The listing builds one solid part. Answer for the finished solid, in the listing's coordinates (mm). A direction names the side the tool comes from. Round coordinates to 2 decimals unless told otherwise and drop trailing zeros. Order: outer loops, then holes, each group sorted by start corner. A loop starts at its lowest first (then second) coordinate and runs counter-clockwise, first axis right, second up. Notation, with made-up numbers: (-22.5, -10) - (-12.5, -10) arc R21 ccw to (-12.5, -6) - close; hole circle Ø6 at (-17.75, -18.75). An arc over 180 degrees is marked (long way). Use CSV: the item, a comma, the result in double quotes. Start each with the question number.
Item 1: Flat-ended cylindrical pins translate along their axes: P1, Ø2, axis at y = 5.5, z = 35.5, coming from the +X side (3 decimals); P2, Ø3.5, axis at y = 0, z = -19.05, coming from the +X side. Find the tip coordinate at first contact, or state that the pin passes through.
Item 2: Determine the mould class of faces 1 (the flat face through (-13, 12.7, 20)), 2 (the flat face through (-20.32, 0, 18)), 3 (the conical face through (-18.66, -0.13, 33.97)), 4 (the flat face through (-13, -12.7, 20)) for opening direction Y: +Y half, -Y half, draft (parallel to the pull), parting line (faces both ways), or undercut.
Item 3: Find section D-D, the plane z = 48.5. Give the vertices of the cut face in (x, y) (3 decimals), plus the area to 3 significant figures.
Item 4: Straight lines are drawn through the part: line 1 along Z through (x, y) = (-12.25, 0); line 2 along Z through (x, y) = (-5.75, 0); line 3 along Z through (x, y) = (-7, 0). For each, find the intervals that lie inside material, in ascending order. Write a range as [from, to].
Item 5: For faces 5 (the flat face through (-3.175, 0, 44)), 6 (the cylindrical face through (-10.515, 0.607, 36.216)), 7 (the flat face through (-11, 0, -25.4)), determine the directions among +Z, -Z, +X, -X, +Y, -Y from which every point of the face is accessible in a straight line to the end or side of a thin tool.
Item 6: Find section B-B, the plane y = -4.25. Give the vertices of the cut face in (x, z) (3 decimals), plus the area to 3 significant figures.
Item 7: Find section C-C, the plane x = -8.75. Give the vertices of the cut face in (y, z), plus the area to 3 significant figures.
Item 8: Find section A-A, the plane x = -12.75. Give the vertices of the cut face in (y, z).
```python
from build123d import *

# Parameters (mm, degrees)
BOSS_EXTRUDE1_DEPTH        = 12.7
SKETCH7_W                  = 1.905
SKETCH7_H                  = 44.45
CUT_EXTRUDE1_DEPTH         = 72.346425278
FILLET1_R                  = 9.525
F_10_32_TAPPED_HOLE1_D     = 4.0386
F_10_32_TAPPED_HOLE1_DEPTH = 14.478
F_10_32_TAPPED_HOLE1_TIP   = 1.213317848
F_10_32_TAPPED_HOLE2_D     = 4.0386
F_10_32_TAPPED_HOLE2_DEPTH = 14.478
F_10_32_TAPPED_HOLE2_TIP   = 1.213317848


with BuildPart() as part:
    # Sketch1 → Boss-Extrude1 (new, symmetric)
    with BuildSketch(Plane(origin=(0, 0, 0), x_dir=(1, 0, 0), z_dir=(0, 1, 0))):
        with BuildLine():
            Line((-1.27, 10.975768811), (-1.27, 25.4))
            Line((-1.27, 25.4), (-20.32, 25.4))
            Line((-20.32, 25.4), (-20.32, -63.5))
            Line((-20.32, -63.5), (-1.27, -63.5))
            Line((-1.27, -63.5), (-1.27, -10.975768811))
            ThreePointArc((-1.27, -10.975768811), (-11.049, 0), (-1.27, 10.975768811))
        make_face()
    extrude(amount=BOSS_EXTRUDE1_DEPTH, both=True)

    # Sketch7 → Cut-Extrude1 (cut, through all)
    with BuildSketch(Plane(origin=(0, 12.7, 0), x_dir=(1, 0, 0), z_dir=(0, 1, 0))):
        with Locations((-2.2225, -41.275)):
            Rectangle(SKETCH7_W, SKETCH7_H)
    extrude(amount=-CUT_EXTRUDE1_DEPTH, mode=Mode.SUBTRACT)

    # Fillet1
    # the kernel refuses this fillet: 9.525 mm, written as the material it adds along each edge
    with BuildSketch(Plane(origin=(-3.175, 12.7, 19.05), x_dir=(1, 0, 0), z_dir=(0, -1, 0))) as fillet1_piece_1:
        with BuildLine():
            CenterArc((9.525, 5.715), FILLET1_R, 180, 36.869897646)
            Line((0, 5.715), (-0.1905, 5.715))
            Line((-0.1905, 5.715), (-0.1905, 0))
            Line((-0.1905, 0), (0, -0.1905))
            ThreePointArc((0, -0.1905), (0.9525, -0.1905), (1.7526, -0.1143))
            Line((1.7526, -0.1143), (1.905, 0))
        make_face()
    extrude(amount=25.4)

    # #10-32 Tapped Hole1
    with Locations(Plane(origin=(-3.175, 0, 0), x_dir=(0, 0, -1), z_dir=(1, 0, 0))):
        with Locations((-53.34, 0), (-34.29, 0)):
            Hole(F_10_32_TAPPED_HOLE1_D / 2, depth=F_10_32_TAPPED_HOLE1_DEPTH)
            with Locations((0, 0, -(F_10_32_TAPPED_HOLE1_DEPTH + F_10_32_TAPPED_HOLE1_TIP / 2))):  # 118° drill point
                Cone(0, F_10_32_TAPPED_HOLE1_D / 2, F_10_32_TAPPED_HOLE1_TIP, mode=Mode.SUBTRACT)

    # #10-32 Tapped Hole2
    with Locations(Plane(origin=(-1.27, 0, 0), x_dir=(0, 0, -1), z_dir=(1, 0, 0))):
        with Locations((19.05, 0)):
            Hole(F_10_32_TAPPED_HOLE2_D / 2, depth=F_10_32_TAPPED_HOLE2_DEPTH)
            with Locations((0, 0, -(F_10_32_TAPPED_HOLE2_DEPTH + F_10_32_TAPPED_HOLE2_TIP / 2))):  # 118° drill point
                Cone(0, F_10_32_TAPPED_HOLE2_D / 2, F_10_32_TAPPED_HOLE2_TIP, mode=Mode.SUBTRACT)


solid = part.part
```
Worked out:
1,P1,"stops at x = -3.175"
1,P2,"stops at x = -15.91"
2,face 1,"+Y half"
2,face 2,"draft"
2,face 3,"undercut"
2,face 4,"-Y half"
3,outline,"(-20.32, -12.7) - (-3.175, -12.7) - (-3.175, 12.7) - (-20.32, 12.7) - close"
3,area,"435 mm²"
4,line 1,"z = [-25.4, -21.07], [-17.03, 32.27], [36.31, 51.32], [55.36, 63.5]"
4,line 2,"z = [-25.4, -21.07], [-17.03, -9.43], [9.43, 32.27], [36.31, 51.32], [55.36, 63.5]"
4,line 3,"z = [-25.4, -21.07], [-17.03, -8.55], [8.55, 32.27], [36.31, 51.32], [55.36, 63.5]"
5,face 5,"+Z, +X, +Y, -Y"
5,face 6,"+X"
5,face 7,"-Z, +X, -X, +Y, -Y"
6,outline,"(-20.32, -25.4) - (-1.27, -25.4) - (-1.27, -10.976) arc R11.049 cw to (-1.27, 10.976) - (-1.27, 19.05) arc R9.525 cw to (-3.175, 24.765) - (-3.175, 63.5) - (-20.32, 63.5) - close"
6,area,"1,450 mm²"
7,outline,"(-12.7, -25.4) - (12.7, -25.4) - (12.7, -6.75) - (-12.7, -6.75) - close; (-12.7, 6.75) - (12.7, 6.75) - (12.7, 63.5) - (-12.7, 63.5) - close; hole circle Ø4.04 at (0, -19.05); hole circle Ø4.04 at (0, 34.29); hole circle Ø4.04 at (0, 53.34)"
7,area,"1,880 mm²"
8,outline,"(-12.7, -25.4) - (12.7, -25.4) - (12.7, 63.5) - (-12.7, 63.5) - close; hole circle Ø4.04 at (0, -19.05); hole circle Ø4.04 at (0, 34.29); hole circle Ø4.04 at (0, 53.34)"
